Part model, mm, in its own coordinate system. Face numbers are marked on the shaded views. A direction names the side the tool comes from. Coordinates: 2 decimals unless noted, no trailing zeros. Loops run counter-clockwise (first coordinate to the right, second up) from the corner with the lowest first, then second, coordinate; pieces in that order, holes last. Notation, with made-up numbers: M 66,45.5 L 90,45.5 A23 ccw 90,62.5 Z; hole C 40.5,23 d1. An arc over 180 degrees is marked long. Use a Markdown table: item, result. Add a question column.
1) Band-saw the part on B-B (y = -0.5). List the corners of the cut face in (x, z), plus the area to 3 significant figures.
2) Pull direction Y, two halves, no side cores. Call the marked faces 1, 2 and 3: released by +Y, released by -Y, zero draft, split by the parting line, or undercut.
3) Tool access for the marked faces 4 and 5: list every direction of +Z, -Z, +X, -X, +Y, -Y with a clear straight run to the whole face (end or side of a thin tool).
4) Band-saw the part on C-C (x = -4.5). List the corners of the cut face in (y, z), plus the area to 3 significant figures.
5) Wall check: probe 1 along X at (y, z) = (9, 10); probe 2 along Y at (x, z) = (7.5, 16.5); probe 3 along X at (y, z) = (4.5, 5). Give the ranges that are in metal, low to high. Write a range as from..to.
6) Pin check, flat tip, straight feed: pin 1 Ø2 at (x, y) = (20, -18) entering from +Z. Stop position of the tip, or through.
7) Band-saw the part on A-A (z = 15). List the corners of the cut face in (x, y).
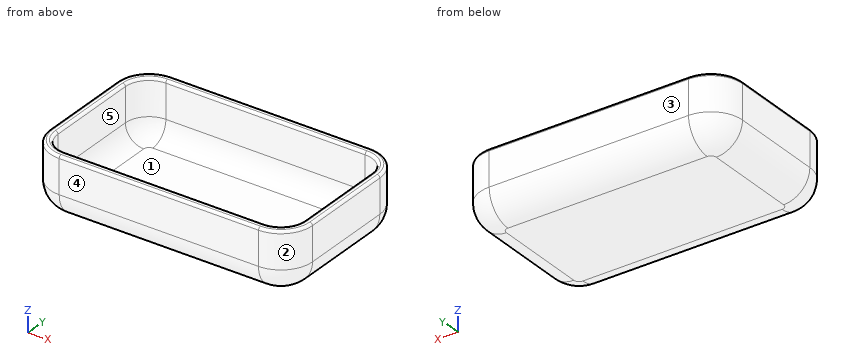
from build123d import *

# Parameters (mm, degrees)
PAD_DEPTH   = 24
FILLET_R    = 10
THICKNESS_T = -3
FILLET001_R = 1


with BuildPart() as part:
    # Sketch (on XY_Plane of Origin) → Pad (new body)
    with BuildSketch(Plane.XY):
        with BuildLine():
            Line((-38, -30), (38, -30))
            ThreePointArc((38, -30), (46.485281, -26.485281), (50, -18))
            Line((50, -18), (50, 18))
            ThreePointArc((50, 18), (46.485281, 26.485281), (38, 30))
            Line((38, 30), (-38, 30))
            ThreePointArc((-38, 30), (-46.485281, 26.485281), (-50, 18))
            Line((-50, 18), (-50, -18))
            ThreePointArc((-50, -18), (-46.485281, -26.485281), (-38, -30))
        make_face()
    extrude(amount=PAD_DEPTH)

    # Fillet
    fillet_edges = [part.edges().sort_by_distance(p)[0] for p in [
        (0, -30, 0),
    ]]
    fillet(fillet_edges, radius=FILLET_R)

    # Thickness
    thickness_openings = [part.faces().sort_by_distance(p)[0] for p in [
        (0, 0, 24),
    ]]
    offset(amount=THICKNESS_T, openings=thickness_openings)

    # Fillet001
    fillet001_edges = [part.edges().sort_by_distance(p)[0] for p in [
        (0, -30, 24),
        (-47, 0, 24),
    ]]
    fillet(fillet001_edges, radius=FILLET001_R)


solid = part.part
Entries:
| question | item | result |
|---|---|---|
| 1 | outline | M -50,10 A10 ccw -40,0 L 40,0 A10 ccw 50,10 L 50,23 A1 ccw 49,24 L 48,24 A1 ccw 47,23 L 47,10 A7 cw 40,3 L -40,3 A7 cw -47,10 L -47,23 A1 ccw -48,24 L -49,24 A1 ccw -50,23 Z |
| 1 | area | 403 mm2 |
| 2 | face 1 | undercut |
| 2 | face 2 | released by -Y |
| 2 | face 3 | released by +Y |
| 3 | face 4 | +Z, -Z, +X, -X, -Y |
| 3 | face 5 | +Z |
| 4 | outline | M -30,10 A10 ccw -20,0 L 20,0 A10 ccw 30,10 L 30,23 A1 ccw 29,24 L 28,24 A1 ccw 27,23 L 27,10 A7 cw 20,3 L -20,3 A7 cw -27,10 L -27,23 A1 ccw -28,24 L -29,24 A1 ccw -30,23 Z |
| 4 | area | 283 mm2 |
| 5 | probe 1 | -50..-47, 47..50 |
| 5 | probe 2 | -30..-27, 27..30 |
| 5 | probe 3 | -48.66..-44.9, 44.9..48.66 |
| 6 | pin 1 | z = 3 |
| 7 | outline | M -50,-18 A12 ccw -38,-30 L 38,-30 A12 ccw 50,-18 L 50,18 A12 ccw 38,30 L -38,30 A12 ccw -50,18 Z; hole M -47,-18 A9 ccw -38,-27 L 38,-27 A9 ccw 47,-18 L 47,18 A9 ccw 38,27 L -38,27 A9 ccw -47,18 Z |
